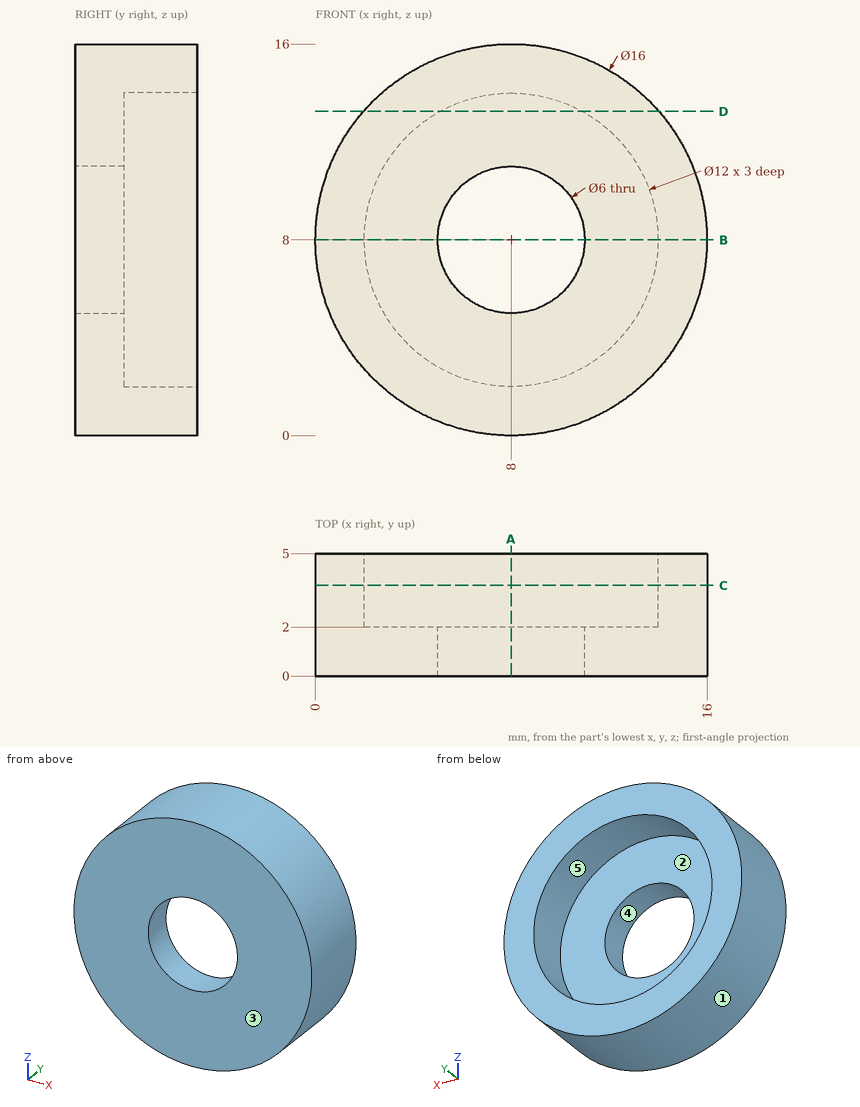
Verification items for this drawing (mm, ordinates from the low corner). A direction names the side the tool comes from. Coordinates: 2 decimals unless noted, no trailing zeros. Write each loop counter-clockwise with the first axis right and the second up, starting at its lowest first coordinate (ties: lowest second). Pieces come first, ordered by that corner, then holes. Notation, with made-up numbers: M 89.25,5.25 L 107.25,5.25 A27 cw 107.25,38.25 Z; hole C -38,-10.5 d3. An arc over 180 degrees is marked long. One line per item, written item: value. Start each with the question number.
(1) Sectioned sample at B-B, the plane z = 8. Enter the section's corners in (x, y), and give its area (3 significant figures).
(2) Sectioned sample at A-A, the plane x = 8. Enter the section's corners in (y, z).
(3) Scan lines: line 1 along X through (y, z) = (3, 8); line 2 along X through (y, z) = (1.2, 8); line 3 along Y through (x, z) = (6, 11.75). Record each from-to range of solid material in increasing order. Write a range as [from, to].
(4) Release check for a two-part mould opening along Z. For the marked faces 1, 2 and 3 record: released by +Z, released by -Z, zero draft, split by the parting line, or undercut.
(5) Sectioned sample at D-D, the plane z = 13.25. Enter the section's corners in (x, y).
(6) Tool access check on the marked faces 4 and 5. Record the directions out of +Z, -Z, +X, -X, +Y, -Y that give a thin tool (end or side, any length) a straight path to the whole face; none if there is none.
(7) Sectioned sample at C-C, the plane y = 3.7. Enter the section's corners in (x, z), and give its area (3 significant figures).
(8) Depth check by flat-ended pin: pin 1 (1.5 mm diameter, centred on y = 3, z = 13, fed in from -X); pin 2 (1.5 mm diameter, centred on x = 2, y = 3.5, fed in from +Z); pin 3 (8 mm diameter, centred on x = 3, z = 8, fed in from -Y); pin 4 (5 mm diameter, centred on x = 8, z = 8, fed in from -Y). Enter the tip coordinate at first touch or a pass-through.
Filled sheet:
1. outline: M 0,0 L 5,0 L 5,2 L 2,2 L 2,5 L 0,5 Z; M 11,0 L 16,0 L 16,5 L 14,5 L 14,2 L 11,2 Z
1. area: 32.0 mm²
2. outline: M 0,0 L 5,0 L 5,2 L 2,2 L 2,5 L 0,5 Z; M 0,11 L 2,11 L 2,14 L 5,14 L 5,16 L 0,16 Z
3. line 1: [0, 2], [14, 16]
3. line 2: [0, 5], [11, 16]
3. line 3: [0, 2]
4. face 1: split by the parting line
4. face 2: undercut
4. face 3: zero draft
5. outline: M 1.96,0 L 14.04,0 L 14.04,5 L 10.9,5 L 10.9,2 L 5.1,2 L 5.1,5 L 1.96,5 Z
6. face 4: +Y, -Y
6. face 5: +Y
7. outline: C 8,8 d16; hole C 8,8 d12
7. area: 88.0 mm²
8. pin 1: x = 1.22
8. pin 2: z = 14.04
8. pin 3: y = 0
8. pin 4: through
